The model under review builds one solid part; all positions refer to its coordinate system, in mm. A direction names the side the tool comes from. Round coordinates to 2 decimals unless told otherwise and drop trailing zeros. Order: outer loops, then holes, each group sorted by start corner. A loop starts at its lowest first (then second) coordinate and runs counter-clockwise, first axis right, second up.
1) Mouldability with a two-part tool opening along Z and no side actions: class faces 1 (the face through (-0.7, 8, 8)), 2 (the face through (16, 9, -1.5)), 3 (the face through (3.7, -6.7, 6)) as pulls with the +Z half, pulls with the -Z half, needs draft (parallel to the pull), parting line crosses it, or undercut.
2) Consider section B-B (x = 8). Give the boundary of the cut face in (y, z).
3) Machinability: for faces 4 (the face through (12, -6.7, 0.2)), 5 (the face through (19, -6.5, 8)), 6 (the face through (15.7, 24, -1.7)), which of the approach directions +Z, -Z, +X, -X, +Y, -Y give a long, thin tool a straight path to every point of the face, cutting with its end or side? Answer none if there is none.
4) Clearance check with a flat-ended pin moving along its axis: P1, Ø9.5, axis at x = 12.5, z = 9.5, coming from the +Y side. State where the tip first meets the part, or that it passes through.
5) Consider section C-C (y = 14.5). Give the boundary of the cut face in (x, z).
6) Consider section D-D (x = 29.5). Give the boundary of the cut face in (y, z), then the cut area to 3 significant figures.
7) To check wall thickness, follow L1, parallel to X at y = 3, z = -1; L2, parallel to Z at x = 29, y = -2.5; L3, parallel to Y at x = 18.5, z = 0. State the ranges of each line that lie inside material, in increasing order.
8) Consider section A-A (z = 2.5). Give the boundary of the cut face in (x, y).
from build123d import *

# Parameters (mm, degrees)
BOX012_W     = 14
BOX012_H     = 10
BOX012_DEPTH = 10
BOX011_W     = 32
BOX011_H     = 35
BOX011_DEPTH = 19
BOX010_W     = 33
BOX010_H     = 31
BOX010_DEPTH = 20
FILLET_R     = 0.3


with BuildPart() as cubo001:
    # Box012 → Box012 (new body)
    with BuildSketch(Plane(origin=(-2, -11, -4), x_dir=(1, 0, 0), z_dir=(0, 0, 1))):
        with Locations((7, 5)):
            Rectangle(BOX012_W, BOX012_H)
    extrude(amount=BOX012_DEPTH)


with BuildPart() as cubo:
    # Box011 → Box011 (new body)
    with BuildSketch(Plane(origin=(-0.2, -6.5, -1.5), x_dir=(1, 0, 0), z_dir=(0, 0, 1))):
        with Locations((16, 17.5)):
            Rectangle(BOX011_W, BOX011_H)
    extrude(amount=BOX011_DEPTH)


with BuildPart() as cut001:
    # Box010 → Box010 (new body)
    with BuildSketch(Plane(origin=(-0.7, -7, -2), x_dir=(1, 0, 0), z_dir=(0, 0, 1))):
        with Locations((16.5, 15.5)):
            Rectangle(BOX010_W, BOX010_H)
    extrude(amount=BOX010_DEPTH)

    # Cut: cut Cubo
    add(cubo.part, mode=Mode.SUBTRACT)

    # Fillet
    fillet_edges = [cut001.edges().sort_by_distance(p)[0] for p in [
        (-0.7, -7, 8),
        (-0.7, 8.5, 18),
        (-0.7, 8.5, -2),
        (15.8, -7, -2),
        (32.3, -7, 8),
        (15.8, -7, 18),
        (32.3, 8.5, 18),
        (32.3, 8.5, -2),
    ]]
    fillet(fillet_edges, radius=FILLET_R)

    # Cut001: cut Cubo001
    add(cubo001.part, mode=Mode.SUBTRACT)


solid = cut001.part
Answer below:
1. face 1: needs draft
1. face 2: undercut
1. face 3: pulls with the -Z half
2. outline: (-7, 6) - (-6.5, 6) - (-6.5, 17.5) - (24, 17.5) - (24, 18) - (-6.7, 18) arc R0.3 ccw to (-7, 17.7) - close; (-1, -2) - (24, -2) - (24, -1.5) - (-1, -1.5) - close
3. face 4: -Z, -X, -Y
3. face 5: +Y
3. face 6: +Z, -Z, +X, -X, +Y
4. P1: stops at y = -6.5
5. outline: (-0.7, -1.7) arc R0.3 ccw to (-0.4, -2) - (32, -2) arc R0.3 ccw to (32.3, -1.7) - (32.3, 17.7) arc R0.3 ccw to (32, 18) - (-0.4, 18) arc R0.3 ccw to (-0.7, 17.7) - close; hole (-0.2, -1.5) - (31.8, -1.5) - (31.8, 17.5) - (-0.2, 17.5) - close
6. outline: (-7, -1.7) arc R0.3 ccw to (-6.7, -2) - (24, -2) - (24, -1.5) - (-6.5, -1.5) - (-6.5, 17.5) - (24, 17.5) - (24, 18) - (-6.7, 18) arc R0.3 ccw to (-7, 17.7) - close
6. area: 40.5 mm2
7. L1: x = -0.7 to -0.2, 31.8 to 32.3
7. L2: z = -2 to -1.5, 17.5 to 18
7. L3: y = -7 to -6.5
8. outline: (-0.7, -1) - (-0.2, -1) - (-0.2, 24) - (-0.7, 24) - close; (12, -7) - (32, -7) arc R0.3 ccw to (32.3, -6.7) - (32.3, 24) - (31.8, 24) - (31.8, -6.5) - (12, -6.5) - close
